Autodesk Inventor part; units mm, degrees
ref_plane "CA3_XY" through (0, 0, -0.4) normal (-1, 0, 0) x (0, 0, -1)
ref_plane "CA3_YZ" through (0, 0, -0.4) normal (0, 0, -1) x (0, -1, 0)
ref_plane "CA3_ZX" through (0, 0, -0.4) normal (0, -1, 0) x (-1, 0, 0)
sketch "__1" plane through (0, 0, 0) normal (0, 0, 1) x (1, 0, 0)
  arc A0 (5.5712, -4.2381) -> (-5.5712, -4.2381) centre (0, 0) ccw
  line L0 (-5.5712, -4.2381) -> (-3.05, -1.7168)
  arc A1 (-3.5, 0) -> (-3.05, -1.7168) centre (0, 0) ccw
  line L1 (-3.5, 0) -> (-5.4, 0)
  arc A2 (-1.8469, 5.0743) -> (-5.4, 0) centre (0, 0) ccw
  line L2 (-1.8469, 5.0743) -> (-1.1971, 3.2889)
  arc A3 (1.1971, 3.2889) -> (-1.1971, 3.2889) centre (0, 0) ccw
  line L3 (1.1971, 3.2889) -> (1.8469, 5.0743)
  arc A4 (5.4, 0) -> (1.8469, 5.0743) centre (0, 0) ccw
  line L4 (5.4, 0) -> (3.5, 0)
  arc A5 (3.05, -1.7168) -> (3.5, 0) centre (0, 0) ccw
  line L5 (3.05, -1.7168) -> (5.5712, -4.2381)
extrude "Extrusion1" add sketch "__1" against normal blind 0.8
ref_plane "CA3_XY" through (0, 0, -0.4) normal (-1, 0, 0) x (0, 0, -1)
ref_plane "CA3_YZ" through (0, 0, -0.4) normal (0, 0, -1) x (0, -1, 0)
ref_plane "CA3_ZX" through (0, 0, -0.4) normal (0, -1, 0) x (-1, 0, 0)
properties part number "METW-7"
The listing builds one solid part. Answer for the finished solid, in the listing's coordinates (mm). A direction names the side the tool comes from. Round coordinates to 2 decimals unless told otherwise and drop trailing zeros. Order: outer loops, then holes, each group sorted by start corner. A loop starts at its lowest first (then second) coordinate and runs counter-clockwise, first axis right, second up. Notation, with made-up numbers: (5, 86.5) - (64, 86.5) arc R9 cw to (64, 98.5) - close; hole circle Ø11 at (20, 43.25). An arc over 180 degrees is marked (long way). Put each result on its own line as item: value. Start each with the question number.
(1) Determine the mould class of faces 3 (the flat face through (-4.328, -2.995, -0.394)), 4 (the cylindrical face through (-4.4, 3.13, -0.39)), 5 (the cylindrical face through (4.45, 3.06, -0.39)), 6 (the flat face through (-1.1, 3.5, -0.8)) for opening direction Y: released by +Y, released by -Y, zero draft, split by the parting line, or undercut.
(2) Straight lines are drawn through the part: probe 1 along X at (y, z) = (1, -0.1); probe 2 along Y at (x, z) = (-4.5, -0.6); probe 3 along X at (y, z) = (2, -0.2). For each, find the intervals that lie inside material, in ascending order. Write a range as from..to.
(3) Find section B-B (z = -0.4). Give the vertices of the cut face in (x, y), plus the area to 3 significant figures.
(4) Find section C-C (x = -4.75). Give the vertices of the cut face in (y, z).
(5) Find section A-A (y = -1.5). Give the vertices of the cut face in (x, z).
(6) Find section D-D (y = 4.5). Give the vertices of the cut face in (x, z), plus the area to 3 significant figures.
(7) For faces 1 (the cylindrical face through (0.218, 6.997, -0.394)), 2 (the flat face through (4.293, -2.96, -0.394)), determine the directions among +Z, -Z, +X, -X, +Y, -Y from which every point of the face is accessible in a straight line to the end or side of a thin tool.
Reply:
1. face 3: released by -Y
1. face 4: undercut
1. face 5: undercut
1. face 6: zero draft
2. probe 1: -6.93..-5.31, 5.31..6.93
2. probe 2: -3.17..0, 2.98..5.36
2. probe 3: -6.71..-5.02, 5.02..6.71
3. outline: (-5.57, -4.24) - (-3.05, -1.72) arc R3.5 cw to (-3.5, 0) - (-5.4, 0) arc R5.4 cw to (-1.85, 5.07) - (-1.2, 3.29) arc R3.5 cw to (1.2, 3.29) - (1.85, 5.07) arc R5.4 cw to (5.4, 0) - (3.5, 0) arc R3.5 cw to (3.05, -1.72) - (5.57, -4.24) arc R7 ccw (long way) to start
3. area: 59.3 mm^2
4. outline: (-3.42, -0.8) - (0, -0.8) - (0, 0) - (-3.42, 0) - close; (2.57, -0.8) - (5.14, -0.8) - (5.14, 0) - (2.57, 0) - close
5. outline: (-6.84, -0.8) - (-3.16, -0.8) - (-3.16, 0) - (-6.84, 0) - close; (3.16, -0.8) - (6.84, -0.8) - (6.84, 0) - (3.16, 0) - close
6. outline: (-5.36, -0.8) - (-2.98, -0.8) - (-2.98, 0) - (-5.36, 0) - close; (-1.64, -0.8) - (1.64, -0.8) - (1.64, 0) - (-1.64, 0) - close; (2.98, -0.8) - (5.36, -0.8) - (5.36, 0) - (2.98, 0) - close
6. area: 6.42 mm^2
7. face 1: +Z, -Z
7. face 2: +Z, -Z, -Y
